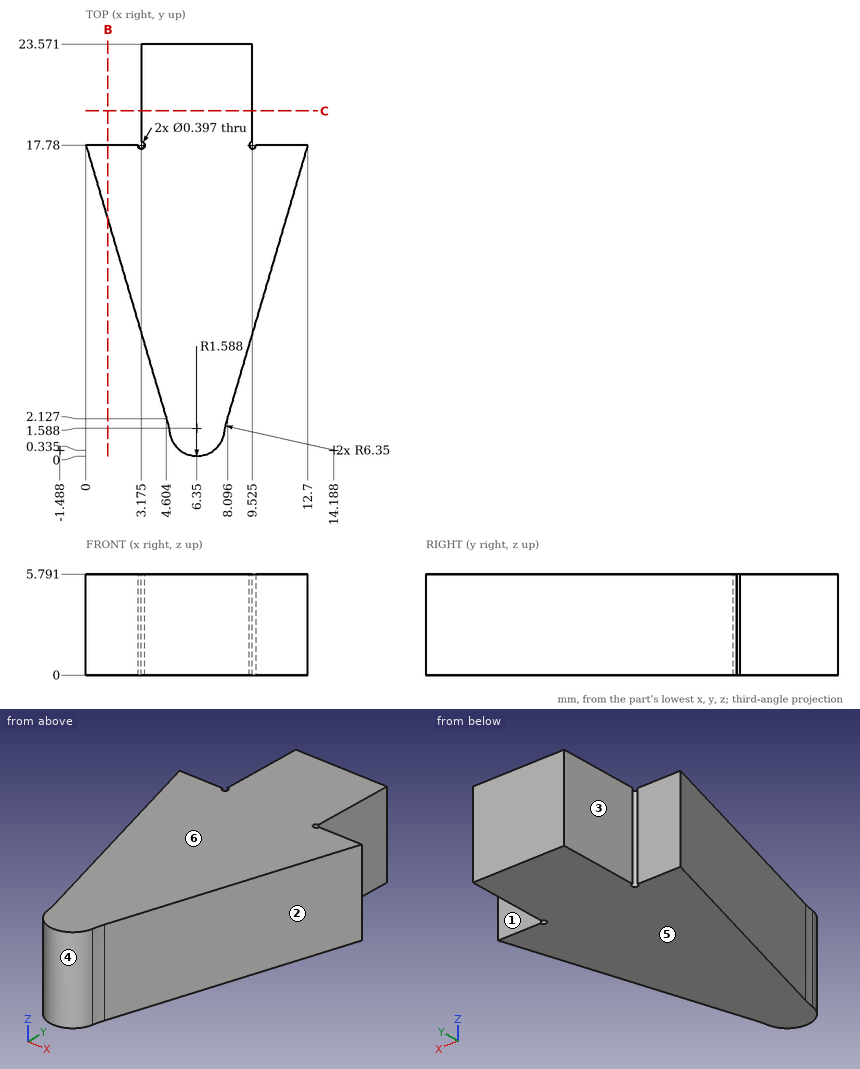
The figure shows three views and two pictorial views of one solid part (mm, origin at its lowest corner). Answer the questions. A direction names the side the tool comes from. Coordinates: 2 decimals unless noted, no trailing zeros. Loops run counter-clockwise (first coordinate to the right, second up) from the corner with the lowest first, then second, coordinate; pieces in that order, holes last. Notation, with made-up numbers: M 27.25,-4 L 82.25,-4 A24 ccw 82.25,34 Z; hole C 55,54 d6. An arc over 180 degrees is marked long. Answer as CSV lines item,"result". Start each with the question number.
(1) Find the intervals of material crossed by L1, parallel to X at y = 19.5, z = 4.75 (1 decimal); L2, parallel to Y at x = 6.5, z = 3.15; L3, parallel to X at y = 14.5, z = 2.65 (1 decimal), in increasing order. Write a range as [from, to].
(2) The part is cut by section B-B (x = 1.25). Give the vertices of the cut face in (y, z), and give its area (3 significant figures).
(3) The part is cut by section C-C (y = 19.75). Give the vertices of the cut face in (x, z) (1 decimal).
(4) Given pin 1 (2.5 mm diameter, centred on x = 1, z = 2, fed in from +Y); pin 2 (1.5 mm diameter, centred on y = 20, z = 3.5, fed in from -X) (1 decimal); pin 3 (1.5 mm diameter, centred on x = 5.5, y = 5, fed in from -Z); pin 4 (1 mm diameter, centred on y = 3.5, z = 1.5, fed in from +X), each flat-ended and moving along its own axis, determine where each tip first touches the part or whether it passes through.
(5) The mould has two halves that part along Z. Classify the marked faces 4, 5 and 6: pulls with the +Z half, pulls with the -Z half, needs draft (parallel to the pull), parting line crosses it, or undercut.
(6) For the marked faces 1, 2 and 3, determine the directions among +Z, -Z, +X, -X, +Y, -Y from which every point of the face is accessible in a straight line to the end or side of a thin tool.
Determined:
1,L1,"[3.2, 9.5]"
1,L2,"[0.01, 23.57]"
1,L3,"[1, 11.7]"
2,outline,"M 13.53,0 L 17.78,0 L 17.78,5.79 L 13.53,5.79 Z"
2,area,"24.6 mm2"
3,outline,"M 3.2,0 L 9.5,0 L 9.5,5.8 L 3.2,5.8 Z"
4,pin 1,"y = 17.78"
4,pin 2,"x = 3.2"
4,pin 3,"z = 0"
4,pin 4,"x = 8.65"
5,face 4,"needs draft"
5,face 5,"pulls with the -Z half"
5,face 6,"pulls with the +Z half"
6,face 1,"+Z, -Z, +X, +Y"
6,face 2,"+Z, -Z, +X, -Y"
6,face 3,"+Z, -Z, -X, +Y"
